Source: CAD feature listing. Evaluate the final solid. Frame: model axes, mm. Give positions to 0.01 mm unless a question says otherwise; leave off trailing zeros. Order: outer loops, then holes, each group sorted by start corner. A loop starts at its lowest first (then second) coordinate and runs counter-clockwise, first axis right, second up. Notation, with made-up numbers: M 80,-2.5 L 106,-2.5 A17 cw 106,12.5 Z; hole C 17,3.25 d11. An arc over 180 degrees is marked long. Use CSV: the item, a comma, the result in double quotes. Start each with the question number.
Item 1: Section query A-A on z = 0. Return loops of the section in (x, y).
Item 2: First-contact query: pin 1 (5 mm diameter, centred on x = 102, y = -404.5, fed in from -Z); pin 2 (6 mm diameter, centred on x = 117.5, y = -721, fed in from +Z); pin 3 (5 mm diameter, centred on x = 49.5, z = -324, fed in from -Y). Flat tips, straight axial feed; report the tip coordinate or a pass-through.
Item 3: Ray query, probe 1 along Y at (x, z) = (177, -642); probe 2 along Y at (x, z) = (164.5, 731); probe 3 along Z at (x, y) = (77, 537). Return the intervals inside material, ascending. Write a range as from..to.
from build123d import *


with BuildPart() as part:
    # Sketch → Revolution (revolve)
    with BuildSketch(Plane.XY):
        with BuildLine():
            Line((250, -976.548789), (250, -1004.92))
            Line((250, -1004.92), (213.710075, -1042.499334))
            ThreePointArc((36.289925, -1042.499334), (125, -1054.92), (213.710075, -1042.499334))
            Line((0, -1004.92), (36.289925, -1042.499334))
            Line((0, -976.548789), (0, -1004.92))
            ThreePointArc((13.19869, -961.657339), (3.77459, -966.599408), (0, -976.548789))
            ThreePointArc((236.80131, -961.657339), (125, -954.92), (13.19869, -961.657339))
            ThreePointArc((250, -976.548789), (246.22541, -966.599408), (236.80131, -961.657339))
        make_face()
    revolve(axis=Axis((0, 0, 0), (1, 0, 0)))


solid = part.part
Verdict:
1,outline,"M 0,-1004.92 L 36.29,-1042.5 A323 ccw 213.71,-1042.5 L 250,-1004.92 L 250,-976.55 A15 ccw 236.8,-961.66 A931 ccw 13.2,-961.66 A15 ccw 0,-976.55 Z; M 0,976.55 A15 ccw 13.2,961.66 A931 ccw 236.8,961.66 A15 ccw 250,976.55 L 250,1004.92 L 213.71,1042.5 A323 ccw 36.29,1042.5 L 0,1004.92 Z"
2,pin 1,"z = -974.45"
2,pin 2,"z = 772.76"
2,pin 3,"y = -995.55"
3,probe 1,"-831.76..-708.86, 708.86..831.76"
3,probe 2,"-757.22..-615.72, 615.72..757.22"
3,probe 3,"-903.84..-791.12, 791.12..903.84"
